Autodesk Inventor part; units mm, degrees
ref_plane "YZ Plane" through (0, 0, 0) normal (1, 0, 0) x (0, 1, 0)
ref_plane "XZ Plane" through (0, 0, 0) normal (0, 1, 0) x (-1, 0, 0)
ref_plane "XY Plane" through (0, 0, 0) normal (0, 0, 1) x (1, 0, 0)
sketch "スケッチ1" plane through (0, 0, 0) normal (0, 1, 0) x (-1, 0, 0)
  line L0 (30, -10) -> (-30, -10)
  line L1 (-30, -10) -> (-30, 10)
  line L2 (-30, 10) -> (30, 10)
  line L3 (30, 10) -> (30, -10)
  line L4 (30, -10) -> (-30, 10) construction
  line L5 (30, 10) -> (-30, -10) construction
  point P0 (0, 0)
  point P1 (0, 0)
  dimension "d0" = 60
  dimension "d1" = 20
extrude "押し出し1" add sketch "スケッチ1" along normal blind 10
sketch "スケッチ3" plane through (0, 0, 0) normal (0, -1, 0) x (1, 0, 0)
  line L0 (30, 5.8) -> (-30, 5.8)
  line L1 (-30, 5.8) -> (-30, -5.8)
  line L2 (-30, -5.8) -> (30, -5.8)
  line L3 (30, -5.8) -> (30, 5.8)
  line L4 (30, 10) -> (30, -10)
  line L5 (-30, -10) -> (-30, 10)
  line L6 (30, 5.8) -> (-30, -5.8) construction
  point P0 (0, 0)
  point P1 (0, 0)
  dimension "d12" = 11.6
extrude "押し出し2" cut sketch "スケッチ3" against normal blind 5
sketch "スケッチ4" plane through (0, 5, 0) normal (0, -1, 0) x (1, 0, 0)
  line L0 (-25, 0) -> (25, 0) construction
  point P0 (0, 0)
  point P1 (0, 0)
  dimension "d15" = 50
hole "穴2" at (-25, 5, 0) at (25, 5, 0) direction (0, 1, 0) diameter 2 depth 0.2 tip angle 118
ref_plane "作業平面1" through (0, 0, 10) normal (-1, 0, 0) x (0, 0, 1)
ref_plane "作業平面2" through (-30, 0, 0) normal (0, 0, 1) x (1, 0, 0)
ref_plane "作業平面3" through (0, 5, 0) normal (0, -1, 0) x (1, 0, 0)
properties part number "forkmount" material "ABS プラスチック"
The listing builds one solid part. Answer for the finished solid, in the listing's coordinates (mm). A direction names the side the tool comes from. Round coordinates to 2 decimals unless told otherwise and drop trailing zeros. Write each loop counter-clockwise with the first axis right and the second up, starting at its lowest first coordinate (ties: lowest second). Pieces come first, ordered by that corner, then holes. Notation, with made-up numbers: (12.5, -12) - (21.5, -12) arc R8 ccw to (21.5, -5) - close; hole circle Ø10 at (27.5, 66.5). An arc over 180 degrees is marked (long way). Use a Markdown table: item, result. Add a question column.
1. A tool of negligible diameter and unlimited length cuts with its end or side. For faces 1 (the face through (0, 5, 0)), 2 (the face through (-30, 6, 0)), from which of +Z, -Z, +X, -X, +Y, -Y can it reach the whole face along a straight path? Write none if from no direction.
2. For a pull along Z with two mould halves and no side action, classify faces 3 (the face through (0, 2, -5.8)), 4 (the face through (30, 6, 0)), 5 (the face through (0, 5, -10)) as +Z half, -Z half, draft (parallel to the pull), parting line (faces both ways), or undercut.
3. Consider line 1 (Z direction, x = -26.5, y = 1.75); line 2 (Y direction, x = -24.5, z = -5); line 3 (Z direction, x = 25, y = 5.15). Determine where each line is inside the solid, lowest interval first.
4. The part is cut by section C-C (z = 2.5). Write down the section's boundary in (x, y), and give its area (3 significant figures).
5. The part is cut by section B-B (x = 16.5). Write down the section's boundary in (y, z), and give its area (3 significant figures).
6. A flat-ended cylindrical pin translates along its axis: P1, Ø9.5, axis at x = 0.5, z = 0, coming from the -Y side. Find the tip coordinate at first contact, or state that the pin passes through.
7. The part is cut by section A-A (y = 1). Write down the section's boundary in (x, z), and give its area (3 significant figures).
Reported:
| question | item | result |
|---|---|---|
| 1 | face 1 | +X, -X, -Y |
| 1 | face 2 | +Z, -Z, -X, +Y, -Y |
| 2 | face 3 | undercut |
| 2 | face 4 | draft |
| 2 | face 5 | -Z half |
| 3 | line 1 | -10 to -5.8, 5.8 to 10 |
| 3 | line 2 | 5 to 10 |
| 3 | line 3 | -10 to -1, 1 to 10 |
| 4 | outline | (-30, 5) - (30, 5) - (30, 10) - (-30, 10) - close |
| 4 | area | 300 mm^2 |
| 5 | outline | (0, -10) - (10, -10) - (10, 10) - (0, 10) - (0, 5.8) - (5, 5.8) - (5, -5.8) - (0, -5.8) - close |
| 5 | area | 142 mm^2 |
| 6 | P1 | y = 5 |
| 7 | outline | (-30, -10) - (30, -10) - (30, -5.8) - (-30, -5.8) - close; (-30, 5.8) - (30, 5.8) - (30, 10) - (-30, 10) - close |
| 7 | area | 504 mm^2 |
